from build123d import *

# Parameters (mm, degrees)
SKETCH1_W                 = 393.7
SKETCH1_H                 = 457.2
PLATE_DEPTH               = 12.7
PATTERN_LINEAR_1136_COUNT = 4
PATTERN_LINEAR_1136_PITCH = 127


with BuildPart() as part:
    # Sketch1 → Plate (new body)
    with BuildSketch(Plane.XY):
        with Locations((196.85, 228.6)):
            Rectangle(SKETCH1_W, SKETCH1_H)
    extrude(amount=PLATE_DEPTH)

    # Sketch3 → Hole (revolve, cut)
    with BuildSketch(Plane(origin=(44.45, 38.1, 12.7), x_dir=(0, -1, 0), z_dir=(1, 0, 0))):
        Polygon((0, 0), (0, 29.215464931), (6.35, 25.4), (6.35, 0), align=None)
    hole = revolve(axis=Axis((44.45, 38.1, 19.05), (0, 0, -1)), mode=Mode.SUBTRACT)

    # Pattern Linear 1136: Hole ×4
    with Locations(*[(0, i * PATTERN_LINEAR_1136_PITCH, 0) for i in range(1, PATTERN_LINEAR_1136_COUNT)]):
        add(hole, mode=Mode.SUBTRACT)

    # 草圖複製排列1: Hole at 3 more places
    with Locations((189.2039, 227.04468, 0), (269.22695, 323.07234, 0), (144.04149, 172.849788, 0)):
        add(hole, mode=Mode.SUBTRACT)

    # 草圖複製排列2: Hole at 4 more places
    with Locations((165, 0, 0), (275, 0, 0), (110, 50, 0), (220, 50, 0)):
        add(hole, mode=Mode.SUBTRACT)


solid = part.part
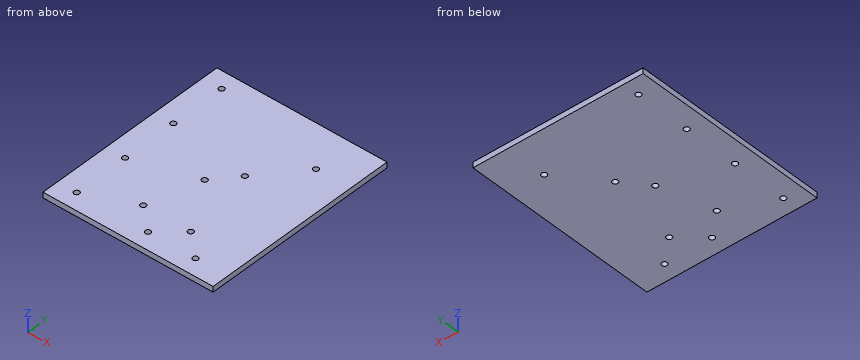
Design review of the part built by this model. Coordinates are the model's own, in mm. Round coordinates to 2 decimals unless told otherwise and drop trailing zeros. Loops run counter-clockwise (first coordinate to the right, second up) from the corner with the lowest first, then second, coordinate; pieces in that order, holes last. Notation, with made-up numbers: M 2.25,-7.75 L 57.25,-7.75 A26 cw 57.25,25.25 Z; hole C -3,49.25 d4. An arc over 180 degrees is marked long. Answer as a JSON object with one key per item and string values.
Item 1: We need section C-C on y = 88.1. Give the boundary of the cut face in (x, z), and give its area (3 significant figures).
Answer sheet:
{"outline": "M 0,0 L 148.1,0 L 148.1,12.7 L 0,12.7 Z; M 160.8,0 L 258.1,0 L 258.1,12.7 L 160.8,12.7 Z; M 270.8,0 L 393.7,0 L 393.7,12.7 L 270.8,12.7 Z", "area": "4,680 mm^2"}
Item 2: We need section A-A on y = 38.1. Give the boundary of the cut face in (x, z), and give its area (3 significant figures).
Answer sheet:
{"outline": "M 0,0 L 38.1,0 L 38.1,12.7 L 0,12.7 Z; M 50.8,0 L 203.1,0 L 203.1,12.7 L 50.8,12.7 Z; M 215.8,0 L 313.1,0 L 313.1,12.7 L 215.8,12.7 Z; M 325.8,0 L 393.7,0 L 393.7,12.7 L 325.8,12.7 Z", "area": "4,520 mm^2"}
Item 3: We need section B-B on x = 209.45. Give the boundary of the cut face in (y, z), and give its area (3 significant figures).
Answer sheet:
{"outline": "M 0,0 L 31.75,0 L 31.75,12.7 L 0,12.7 Z; M 44.45,0 L 457.2,0 L 457.2,12.7 L 44.45,12.7 Z", "area": "5,650 mm^2"}
Item 4: We need section D-D on y = 165.1. Give the boundary of the cut face in (x, z).
Answer sheet:
{"outline": "M 0,0 L 38.1,0 L 38.1,12.7 L 0,12.7 Z; M 50.8,0 L 393.7,0 L 393.7,12.7 L 50.8,12.7 Z"}
Item 5: Wall thickness on L1, parallel to X at y = 88.1, z = 7.25; L2, parallel to X at y = 38.1, z = 7.5; L3, parallel to Y at x = 155, z = 9: over which ranges is each line inside the solid? List them lowest first. Write a range as from..to.
Answer sheet:
{"L1": "x = 0..148.1, 160.8..258.1, 270.8..393.7", "L2": "x = 0..38.1, 50.8..203.1, 215.8..313.1, 325.8..393.7", "L3": "y = 0..81.77, 94.43..457.2"}
